```python
from build123d import *

# Parameters (mm, degrees)
F0_W     = 139.7
F0_H     = 76.2
F0_W_2   = 33.02
F0_H_2   = 3.048
F0_W_3   = 77.47
F1_DEPTH = 76.2
F3_DEPTH = 3.81
F4_DEPTH = 139.701


with BuildPart() as f1:
    # F0 (on Top) → F1 (new body)
    with BuildSketch(Plane.XY):
        Rectangle(F0_W, F0_H)
        with BuildLine():
            ThreePointArc((-63.394407, -18.25625), (-61.534535, -13.766122), (-57.044407, -11.90625))
            Line((-57.044407, -11.90625), (-21.695593, -11.90625))
            ThreePointArc((-21.695593, -11.90625), (-17.205465, -13.766122), (-15.345593, -18.25625))
            Line((-15.345593, -18.25625), (-15.345593, -19.84375))
            ThreePointArc((-15.345593, -19.84375), (-17.205465, -24.333878), (-21.695593, -26.19375))
            Line((-21.695593, -26.19375), (-57.044407, -26.19375))
            ThreePointArc((-57.044407, -26.19375), (-61.534535, -24.333878), (-63.394407, -19.84375))
            Line((-63.394407, -19.84375), (-63.394407, -18.25625))
        make_face(mode=Mode.SUBTRACT)
        with BuildLine():
            ThreePointArc((1.27, -14.605), (3.129872, -10.114872), (7.62, -8.255))
            Line((7.62, -8.255), (25.4, -8.255))
            ThreePointArc((25.4, -8.255), (29.890128, -10.114872), (31.75, -14.605))
            Line((31.75, -14.605), (31.75, -20.955))
            ThreePointArc((31.75, -20.955), (29.890128, -25.445128), (25.4, -27.305))
            Line((25.4, -27.305), (7.62, -27.305))
            ThreePointArc((7.62, -27.305), (3.129872, -25.445128), (1.27, -20.955))
            Line((1.27, -20.955), (1.27, -14.605))
        make_face(mode=Mode.SUBTRACT)
        with BuildLine():
            ThreePointArc((42.545, -15.24), (43.660923, -12.545923), (46.355, -11.43))
            Line((46.355, -11.43), (57.785, -11.43))
            ThreePointArc((57.785, -11.43), (60.479077, -12.545923), (61.595, -15.24))
            Line((61.595, -15.24), (61.595, -20.32))
            ThreePointArc((61.595, -20.32), (60.479077, -23.014077), (57.785, -24.13))
            Line((57.785, -24.13), (46.355, -24.13))
            ThreePointArc((46.355, -24.13), (43.660923, -23.014077), (42.545, -20.32))
            Line((42.545, -20.32), (42.545, -15.24))
        make_face(mode=Mode.SUBTRACT)
        with BuildLine():
            ThreePointArc((-63.394407, 0.79375), (-61.534535, 5.283878), (-57.044407, 7.14375))
            Line((-57.044407, 7.14375), (-21.695593, 7.14375))
            ThreePointArc((-21.695593, 7.14375), (-17.205465, 5.283878), (-15.345593, 0.79375))
            Line((-15.345593, 0.79375), (-15.345593, -0.79375))
            ThreePointArc((-15.345593, -0.79375), (-17.205465, -5.283878), (-21.695593, -7.14375))
            Line((-21.695593, -7.14375), (-57.044407, -7.14375))
            ThreePointArc((-57.044407, -7.14375), (-61.534535, -5.283878), (-63.394407, -0.79375))
            Line((-63.394407, -0.79375), (-63.394407, 0.79375))
        make_face(mode=Mode.SUBTRACT)
        with BuildLine():
            ThreePointArc((-64.134793, 19.84375), (-62.274921, 24.333878), (-57.784793, 26.19375))
            Line((-57.784793, 26.19375), (-20.955207, 26.19375))
            ThreePointArc((-20.955207, 26.19375), (-16.465079, 24.333878), (-14.605207, 19.84375))
            Line((-14.605207, 19.84375), (-14.605207, 18.25625))
            ThreePointArc((-14.605207, 18.25625), (-16.465079, 13.766122), (-20.955207, 11.90625))
            Line((-20.955207, 11.90625), (-57.784793, 11.90625))
            ThreePointArc((-57.784793, 11.90625), (-62.274921, 13.766122), (-64.134793, 18.25625))
            Line((-64.134793, 18.25625), (-64.134793, 19.84375))
        make_face(mode=Mode.SUBTRACT)
        with Locations((31.75, 7.62)):
            Rectangle(F0_W_2, F0_H_2, mode=Mode.SUBTRACT)
        with Locations((27.94, 25.4)):
            Rectangle(F0_W_3, F0_H_2, mode=Mode.SUBTRACT)
    extrude(amount=F1_DEPTH)

    # F0 (on Top) → F3 (join)
    with BuildSketch(Plane.XY):
        with BuildLine():
            Line((-20.955207, 26.19375), (-57.784793, 26.19375))
            ThreePointArc((-57.784793, 26.19375), (-62.274921, 24.333878), (-64.134793, 19.84375))
            Line((-64.134793, 19.84375), (-64.134793, 18.25625))
            ThreePointArc((-64.134793, 18.25625), (-62.274921, 13.766122), (-57.784793, 11.90625))
            Line((-57.784793, 11.90625), (-20.955207, 11.90625))
            ThreePointArc((-20.955207, 11.90625), (-16.465079, 13.766122), (-14.605207, 18.25625))
            Line((-14.605207, 18.25625), (-14.605207, 19.84375))
            ThreePointArc((-14.605207, 19.84375), (-16.465079, 24.333878), (-20.955207, 26.19375))
        make_face()
        with BuildLine():
            Line((-21.695593, 7.14375), (-57.044407, 7.14375))
            ThreePointArc((-57.044407, 7.14375), (-61.534535, 5.283878), (-63.394407, 0.79375))
            Line((-63.394407, 0.79375), (-63.394407, -0.79375))
            ThreePointArc((-63.394407, -0.79375), (-61.534535, -5.283878), (-57.044407, -7.14375))
            Line((-57.044407, -7.14375), (-21.695593, -7.14375))
            ThreePointArc((-21.695593, -7.14375), (-17.205465, -5.283878), (-15.345593, -0.79375))
            Line((-15.345593, -0.79375), (-15.345593, 0.79375))
            ThreePointArc((-15.345593, 0.79375), (-17.205465, 5.283878), (-21.695593, 7.14375))
        make_face()
        with BuildLine():
            Line((-21.695593, -11.90625), (-57.044407, -11.90625))
            ThreePointArc((-57.044407, -11.90625), (-61.534535, -13.766122), (-63.394407, -18.25625))
            Line((-63.394407, -18.25625), (-63.394407, -19.84375))
            ThreePointArc((-63.394407, -19.84375), (-61.534535, -24.333878), (-57.044407, -26.19375))
            Line((-57.044407, -26.19375), (-21.695593, -26.19375))
            ThreePointArc((-21.695593, -26.19375), (-17.205465, -24.333878), (-15.345593, -19.84375))
            Line((-15.345593, -19.84375), (-15.345593, -18.25625))
            ThreePointArc((-15.345593, -18.25625), (-17.205465, -13.766122), (-21.695593, -11.90625))
        make_face()
        with BuildLine():
            Line((25.4, -8.255), (7.62, -8.255))
            ThreePointArc((7.62, -8.255), (3.129872, -10.114872), (1.27, -14.605))
            Line((1.27, -14.605), (1.27, -20.955))
            ThreePointArc((1.27, -20.955), (3.129872, -25.445128), (7.62, -27.305))
            Line((7.62, -27.305), (25.4, -27.305))
            ThreePointArc((25.4, -27.305), (29.890128, -25.445128), (31.75, -20.955))
            Line((31.75, -20.955), (31.75, -14.605))
            ThreePointArc((31.75, -14.605), (29.890128, -10.114872), (25.4, -8.255))
        make_face()
        with BuildLine():
            Line((57.785, -11.43), (46.355, -11.43))
            ThreePointArc((46.355, -11.43), (43.660923, -12.545923), (42.545, -15.24))
            Line((42.545, -15.24), (42.545, -20.32))
            ThreePointArc((42.545, -20.32), (43.660923, -23.014077), (46.355, -24.13))
            Line((46.355, -24.13), (57.785, -24.13))
            ThreePointArc((57.785, -24.13), (60.479077, -23.014077), (61.595, -20.32))
            Line((61.595, -20.32), (61.595, -15.24))
            ThreePointArc((61.595, -15.24), (60.479077, -12.545923), (57.785, -11.43))
        make_face()
        with Locations((31.75, 7.62)):
            Rectangle(F0_W_2, F0_H_2)
        with Locations((27.94, 25.4)):
            Rectangle(F0_W_3, F0_H_2)
    extrude(amount=F3_DEPTH)

    # F2 (on face) → F4 (cut, through all)
    with BuildSketch(Plane(origin=(-69.85, 0, 0), x_dir=(0, -1, 0), z_dir=(-1, 0, 0))):
        Polygon((-38.1, 76.2), (-38.1, 66.954948), (38.1, 49.710575), (38.1, 76.2), align=None)
    extrude(amount=-F4_DEPTH, mode=Mode.SUBTRACT)


solid = f1.part
```
Can you work these out from the model? Positions are in its coordinate system, mm. Coordinates: 2 decimals unless noted, no trailing zeros. Loops run counter-clockwise (first coordinate to the right, second up) from the corner with the lowest first, then second, coordinate; pieces in that order, holes last. Notation, with made-up numbers: (23, 38.5) - (82, 38.5) arc R25 cw to (82, 50.5) - close; hole circle Ø8 at (-34.5, -14.75). An arc over 180 degrees is marked (long way). Answer as CSV lines item,"result". Start each with the question number.
1) Suppose I cut it at A-A (x = -5.5). Please give me the cut outline in (y, z), plus the area to 3 significant figures.
2) Suppose I cut it at C-C (x = -41). Please give me the cut outline in (y, z) (3 decimals).
3) Suppose I cut it at D-D (y = 22). Please give me the cut outline in (x, z), plus the area to 3 significant figures.
4) Suppose I cut it at B-B (z = 19). Count the separate pieces of the cut face and the enclosed holes in it, plus the area to 3 significant figures.
5) Thinking about a two-plate mould opening in Y: for faces 1 (the flat face through (-39, -7.144, 30)), 2 (the flat face through (-1, 38.1, 33)), which applies, pulls with the +Y half, pulls with the -Y half, needs draft (parallel to the pull), parting line crosses it, or undercut?
6) I need wall thicknesses on line 1 (Y direction, x = -27, z = 46); line 2 (Y direction, x = 8.5, z = 22) (3 decimals); line 3 (Y direction, x = 58, z = 20). Which ranges of each line are inside material? Lowest first, please. Write a range as from..to.
7) For pin 1 (4.5 mm diameter, centred on x = -51, y = -16.5, fed in from +Z); pin 2 (3.5 mm diameter, centred on x = 21, y = 26, fed in from +Z); pin 3 (10 mm diameter, centred on x = 51, y = -21, fed in from +Z), each with a flat end and sliding along its axis, tell me the tip position at first contact or that it passes through.
Check result:
1,outline,"(-38.1, 0) - (38.1, 0) - (38.1, 66.95) - (26.92, 64.43) - (26.92, 3.81) - (23.88, 3.81) - (23.88, 63.74) - (-38.1, 49.71) - close"
1,area,"4,260 mm²"
2,outline,"(-38.1, 0) - (38.1, 0) - (38.1, 66.955) - (26.194, 64.261) - (26.194, 3.81) - (11.906, 3.81) - (11.906, 61.027) - (7.144, 59.949) - (7.144, 3.81) - (-7.144, 3.81) - (-7.144, 56.716) - (-11.906, 55.638) - (-11.906, 3.81) - (-26.194, 3.81) - (-26.194, 52.405) - (-38.1, 49.711) - close"
3,outline,"(-69.85, 0) - (69.85, 0) - (69.85, 63.31) - (-14.98, 63.31) - (-14.98, 3.81) - (-63.76, 3.81) - (-63.76, 63.31) - (-69.85, 63.31) - close"
3,area,"5,940 mm²"
4,separate pieces,"1"
4,enclosed holes,"7"
4,area,"7,560 mm²"
5,face 1,"undercut"
5,face 2,"pulls with the +Y half"
6,line 1,"y = -38.1..-26.19, -11.91..-7.14, 7.14..11.91, 26.19..38.1"
6,line 2,"y = -38.1..-27.305, -8.255..23.876, 26.924..38.1"
6,line 3,"y = -38.1..-24.12, -11.44..23.88, 26.92..38.1"
7,pin 1,"stops at z = 3.81"
7,pin 2,"stops at z = 64.61"
7,pin 3,"stops at z = 52.87"
